from build123d import *

# Parameters (mm, degrees)
F1_DEPTH  = 35
F3_DEPTH  = 5
F8_R      = 12.5
F6_R      = 7.5
F10_R     = 3
F11_R     = 4
F12_DEPTH = 5
F13_R     = 4
F14_DEPTH = 5
F15_R     = 3
F16_R     = 5
F17_R     = 5


with BuildPart() as f1:
    # F0 (on Front) → F1 (new body, symmetric)
    with BuildSketch(Plane.XZ):
        with BuildLine():
            Line((-20.25, 15.25), (-20.25, -20.25))
            Line((-20.25, -20.25), (20.25, -20.25))
            Line((20.25, -20.25), (20.25, 15.25))
            ThreePointArc((20.25, 15.25), (18.7855339059, 18.7855339059), (15.25, 20.25))
            Line((15.25, 20.25), (-15.25, 20.25))
            ThreePointArc((-15.25, 20.25), (-18.7855339059, 18.7855339059), (-20.25, 15.25))
        make_face()
        with BuildLine():
            Line((12.25, -15.25), (-12.25, -15.25))
            ThreePointArc((-12.25, -15.25), (-14.3713203436, -14.3713203436), (-15.25, -12.25))
            Line((-15.25, -12.25), (-15.25, 12.25))
            ThreePointArc((-15.25, 12.25), (-14.3713203436, 14.3713203436), (-12.25, 15.25))
            Line((-12.25, 15.25), (12.25, 15.25))
            ThreePointArc((12.25, 15.25), (14.3713203436, 14.3713203436), (15.25, 12.25))
            Line((15.25, 12.25), (15.25, -12.25))
            ThreePointArc((15.25, -12.25), (14.3713203436, -14.3713203436), (12.25, -15.25))
        make_face(mode=Mode.SUBTRACT)
    extrude(amount=F1_DEPTH, both=True)

    # F2 (on face) → F3 (cut, through all)
    with BuildSketch(Plane.XY.offset(20.25)):
        Polygon((6.6, -3.8105117767), (6.6, 3.8105117767), (0, 7.6210235533), (-6.6, 3.8105117767), (-6.6, -3.8105117767), (0, -7.6210235533), align=None)
    extrude(amount=-F3_DEPTH, mode=Mode.SUBTRACT)

    # F8 (on offset) → F9 section 0
    with BuildSketch(Plane.XY.offset(20.25)):
        Circle(F8_R)
    # F6 (on offset) → F9 section 1
    with BuildSketch(Plane.XY.offset(25.25)):
        Circle(F6_R)
    loft()

    # F10
    f10_edges = [f1.edges().sort_by_distance(p)[0] for p in [
        (-12.5, 0, 20.25),
        (-7.5, 0, 25.25),
    ]]
    fillet(f10_edges, radius=F10_R)

    # F11 (on face) → F12 (cut, through all)
    with BuildSketch(Plane.XY.offset(25.25)):
        Circle(F11_R)
    extrude(amount=-F12_DEPTH, mode=Mode.SUBTRACT)

    # F13 (on face) → F14 (join)
    with BuildSketch(Plane(origin=(0, 0, -20.25), x_dir=(1, 0, 0), z_dir=(0, 0, -1))):
        Polygon((-44.4906626391, 2.3624008838), (-43.7589633962, -4.5992523838), (-43.0272641533, -11.5609056514), (-7.9591781516, -19.9412006447), (11.9312597558, -17.8506313793), (43.9934016914, -2.4146651154), (43.2617024485, 4.5469881521), (42.5300032056, 11.5086414197), (7.9591781516, 19.9412006447), (-11.9312597558, 17.8506313793), align=None)
        with Locations((-33.3164834948, -3.5017035195)):
            Circle(F13_R, mode=Mode.SUBTRACT)
        with Locations((33.3164834948, 3.5017035195)):
            Circle(F13_R, mode=Mode.SUBTRACT)
    extrude(amount=F14_DEPTH)

    # F15
    f15_edges = [f1.edges().sort_by_distance(p)[0] for p in [
        (42.530003, -11.508641, -22.75),
        (7.959178, -19.941201, -22.75),
        (-11.93126, -17.850631, -22.75),
        (-44.490663, -2.362401, -22.75),
        (-43.027264, 11.560906, -22.75),
        (-7.959178, 19.941201, -22.75),
        (11.93126, 17.850631, -22.75),
        (43.993402, 2.414665, -22.75),
    ]]
    fillet(f15_edges, radius=F15_R)

    # F16
    f16_edges = [f1.edges().sort_by_distance(p)[0] for p in [
        (-20.25, 1.55528, -20.25),
        (20.25, -1.548771, -20.25),
    ]]
    fillet(f16_edges, radius=F16_R)

    # F17
    f17_edges = [f1.edges().sort_by_distance(p)[0] for p in [
        (-20.25, 26.002018, -20.25),
        (-20.25, -24.446739, -20.25),
        (20.25, 24.422833, -20.25),
        (20.25, -25.971604, -20.25),
    ]]
    fillet(f17_edges, radius=F17_R)


solid = f1.part
Read the model definition and answer for the solid it produces. Units are mm, in the model's axes. A direction names the side the tool comes from. Give positions to 0.01 mm unless a question says otherwise; leave off trailing zeros. Write each loop counter-clockwise with the first axis right and the second up, starting at its lowest first coordinate (ties: lowest second). Pieces come first, ordered by that corner, then holes. Notation, with made-up numbers: (45, -15.75) - (72, -15.75) arc R5 ccw to (72, -9.75) - close; hole circle Ø2 at (39.5, 66). An arc over 180 degrees is marked (long way). Answer in a Markdown table with one row per item. Add a question column.
Item 1: Find the intervals of material crossed by L1, parallel to X at y = 6.5, z = -2.5; L2, parallel to Z at x = -10, y = -9.5, in increasing order.
Item 2: Flat-ended cylindrical pins translate along their axes: P1, Ø2, axis at y = 7.5, z = -17, coming from the -X side; P2, Ø1.5, axis at y = -0.5, z = 18.5, coming from the -X side; P3, Ø8, axis at y = -4, z = 4, coming from the -X side; P4, Ø7, axis at x = -33.32, y = 3.5, coming from the +Z side. Find the tip coordinate at first contact, or state that the pin passes through.
Item 3: Section C-C, the plane x = 36 is taken. Write down the section's boundary in (y, z).
Item 4: Section B-B, the plane y = 26 is taken. Write down the section's boundary in (x, z).
Item 5: Section D-D, the plane z = 17 is taken. Write down the section's boundary in (x, y).
Item 6: Determine the mould class of faces 1 (the face through (-3.346, -5.689, 17.785)), 2 (the face through (-43.766, 4.531, -22.715)), 3 (the face through (14, 0, 20.25)) for opening direction Y: pulls with the +Y half, pulls with the -Y half, needs draft (parallel to the pull), parting line crosses it, or undercut.
Item 7: A tool of negligible diameter and unlimited length cuts with its end or side. For faces 4 (the face through (32, 1, -20.25)), 5 (the face through (-27.273, -10.553, -22.402)), 6 (the face through (-14.39, -0.49, 14.35)), from which of +Z, -Z, +X, -X, +Y, -Y can it reach the whole face along a straight path? Write none if from no direction.
Item 8: Section A-A, the plane z = -7 is taken. Write down the section's boundary in (x, y).
Recorded:
| question | item | result |
|---|---|---|
| 1 | L1 | x = -20.25 to -15.25, 15.25 to 20.25 |
| 1 | L2 | z = -25.25 to -15.25, 15.25 to 20.25 |
| 2 | P1 | stops at x = -21.07 |
| 2 | P2 | stops at x = -19.58 |
| 2 | P3 | stops at x = -20.25 |
| 2 | P4 | passes through |
| 3 | outline | (-13.1, -25.25) - (-6.47, -25.25) - (-6.47, -20.25) - (-13.1, -20.25) - close; (-0.54, -25.25) - (6.26, -25.25) - (6.26, -20.25) - (-0.54, -20.25) - close |
| 4 | outline | (-20.25, -15.25) arc R5 ccw to (-15.25, -20.25) - (15.25, -20.25) arc R5 ccw to (20.25, -15.25) - (20.25, 15.25) arc R5 ccw to (15.25, 20.25) - (-15.25, 20.25) arc R5 ccw to (-20.25, 15.25) - close; hole (-15.25, -12.25) arc R3 ccw to (-12.25, -15.25) - (12.25, -15.25) arc R3 ccw to (15.25, -12.25) - (15.25, 12.25) arc R3 ccw to (12.25, 15.25) - (-12.25, 15.25) arc R3 ccw to (-15.25, 12.25) - close |
| 5 | outline | (-19.93, -35) - (19.93, -35) - (19.93, 35) - (-19.93, 35) - close; hole (-6.6, -3.81) - (0, -7.62) - (6.6, -3.81) - (6.6, 3.81) - (0, 7.62) - (-6.6, 3.81) - close |
| 6 | face 1 | undercut |
| 6 | face 2 | pulls with the +Y half |
| 6 | face 3 | needs draft |
| 7 | face 4 | +Z, +X, +Y, -Y |
| 7 | face 5 | -Z, -X, -Y |
| 7 | face 6 | +Y, -Y |
| 8 | outline | (-20.25, -35) - (-15.25, -35) - (-15.25, 35) - (-20.25, 35) - close; (15.25, -35) - (20.25, -35) - (20.25, 35) - (15.25, 35) - close |
